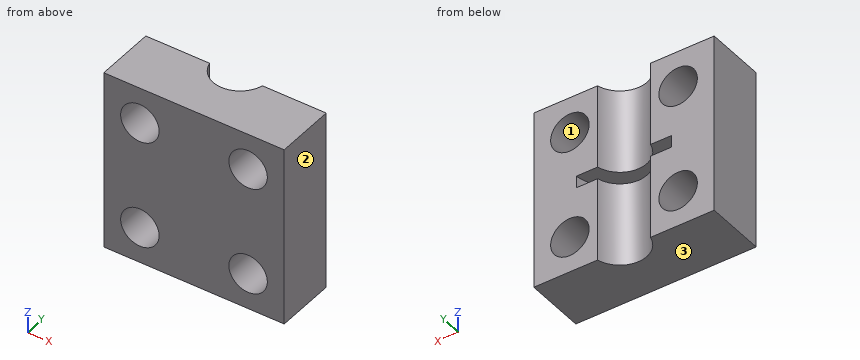
```python
from build123d import *

# Parameters (mm, degrees)
SKIZZE1_W                       = 15
SKIZZE1_H                       = 15
SKIZZE1_R                       = 1.6
AUFSATZ_LINEAR_AUSTRAGEN1_DEPTH = 5
SKIZZE2_R                       = 2.25
SCHNITT_LINEAR_AUSTRAGEN1_DEPTH = 16
SKIZZE3_R                       = 4
SCHNITT_LINEAR_AUSTRAGEN2_DEPTH = 1


with BuildPart() as part:
    # Skizze1 → Aufsatz-Linear austragen1 (new body)
    with BuildSketch(Plane(origin=(0, 0, 0), x_dir=(1, 0, 0), z_dir=(0, 1, 0))):
        Rectangle(SKIZZE1_W, SKIZZE1_H)
        with Locations((-4.5, 4.5)):
            Circle(SKIZZE1_R, mode=Mode.SUBTRACT)
        with Locations((-4.5, -4.5)):
            Circle(SKIZZE1_R, mode=Mode.SUBTRACT)
        with Locations((4.5, -4.5)):
            Circle(SKIZZE1_R, mode=Mode.SUBTRACT)
        with Locations((4.5, 4.5)):
            Circle(SKIZZE1_R, mode=Mode.SUBTRACT)
    extrude(amount=AUFSATZ_LINEAR_AUSTRAGEN1_DEPTH)

    # Skizze2 → Schnitt-Linear austragen1 (cut, through all)
    with BuildSketch(Plane.XY.offset(7.5)):
        with Locations((0, 5.5)):
            Circle(SKIZZE2_R)
    extrude(amount=-SCHNITT_LINEAR_AUSTRAGEN1_DEPTH, mode=Mode.SUBTRACT)

    # Skizze3 → Schnitt-Linear austragen2 (cut)
    with BuildSketch(Plane.XY.offset(0.5)):
        with Locations((0, 5.5)):
            Circle(SKIZZE3_R)
    extrude(amount=-SCHNITT_LINEAR_AUSTRAGEN2_DEPTH, mode=Mode.SUBTRACT)


solid = part.part
```
For this review, take the finished solid that the model builds, in its own axes (mm). Face numbers are marked on the shaded views. Give positions to 0.01 mm unless a question says otherwise; leave off trailing zeros. Loops run counter-clockwise (first coordinate to the right, second up) from the corner with the lowest first, then second, coordinate; pieces in that order, holes last. Notation, with made-up numbers: M 84.5,-13 L 98.5,-13 A32 cw 98.5,18 Z; hole C -30.75,55 d1. An arc over 180 degrees is marked long. One line per item, written item: value. Start each with the question number.
Q1. Add section B-B (y = 4.7). Give the boundary of the cut face in (x, z), and give its area (3 significant figures).
Q2. Draft analysis for pull direction Z (two halves, no side actions). For the marked faces 1, 2 and 3, state which applies: released by +Z, released by -Z, zero draft, split by the parting line, or undercut.
Q3. For L1, parallel to X at y = 3.05, z = 4.5; L2, parallel to Z at x = 0, y = 2.1, list the stretches that pass through material, from the lowest coordinate up.
Q4. Add section C-C (x = -5). Give the boundary of the cut face in (y, z), and give its area (3 significant figures).
Q5. Add section D-D (z = 0). Give the boundary of the cut face in (x, y), and give its area (3 significant figures).
Q6. Add section A-A (z = -4.5). Give the boundary of the cut face in (x, y), and give its area (3 significant figures).
Reply:
1. outline: M -7.5,-7.5 L -2.1,-7.5 L -2.1,-0.5 L -3.92,-0.5 L -3.92,0.5 L -2.1,0.5 L -2.1,7.5 L -7.5,7.5 Z; M 2.1,-7.5 L 7.5,-7.5 L 7.5,7.5 L 2.1,7.5 L 2.1,0.5 L 3.92,0.5 L 3.92,-0.5 L 2.1,-0.5 Z; hole C -4.5,-4.5 d3.2; hole C -4.5,4.5 d3.2; hole C 4.5,-4.5 d3.2; hole C 4.5,4.5 d3.2
1. area: 126 mm²
2. face 1: undercut
2. face 2: zero draft
2. face 3: released by -Z
3. L1: -7.5 to -6.1, -2.9 to 2.9, 6.1 to 7.5
3. L2: -7.5 to -0.5, 0.5 to 7.5
4. outline: M 0,-7.5 L 5,-7.5 L 5,-6.02 L 0,-6.02 Z; M 0,-2.98 L 5,-2.98 L 5,2.98 L 0,2.98 Z; M 0,6.02 L 5,6.02 L 5,7.5 L 0,7.5 Z
4. area: 44.6 mm²
5. outline: M -7.5,0 L 7.5,0 L 7.5,5 L 3.97,5 A4 cw -3.97,5 L -7.5,5 Z
5. area: 53.9 mm²
6. outline: M -7.5,0 L -6.1,0 L -6.1,5 L -7.5,5 Z; M -2.9,0 L 2.9,0 L 2.9,5 L 2.19,5 A2.25 cw -2.19,5 L -2.9,5 Z; M 6.1,0 L 7.5,0 L 7.5,5 L 6.1,5 Z
6. area: 37.3 mm²
